Model file for the job. Use its own axes, mm. A direction names the side the tool comes from. Give positions to 0.01 mm unless a question says otherwise; leave off trailing zeros. Loops run counter-clockwise (first coordinate to the right, second up) from the corner with the lowest first, then second, coordinate; pieces in that order, holes last. Notation, with made-up numbers: M 75.25,-37.5 L 84.25,-37.5 A32 cw 84.25,-1.5 Z; hole C 19.25,46 d2. An arc over 180 degrees is marked long. Answer in a Markdown table with one row per item.
Autodesk Inventor part; units mm, degrees
ref_plane "YZ Plane" through (0, 0, 0) normal (1, 0, 0) x (0, 1, 0)
ref_plane "XZ Plane" through (0, 0, 0) normal (0, 1, 0) x (-1, 0, 0)
ref_plane "XY Plane" through (0, 0, 0) normal (0, 0, 1) x (1, 0, 0)
sketch "スケッチ1" plane through (0, 0, 0) normal (0, 1, 0) x (-1, 0, 0)
  line L0 (12.5, 12.5) -> (-12.5, 12.5)
  line L1 (-12.5, 12.5) -> (-12.5, -12.5)
  line L2 (-12.5, -12.5) -> (12.5, -12.5)
  line L3 (12.5, -12.5) -> (12.5, 12.5)
  line L4 (12.5, 12.5) -> (-12.5, -12.5) construction
  line L5 (-12.5, 12.5) -> (12.5, -12.5) construction
  point P0 (0, 0)
  dimension "d0" = 25
  dimension "d1" = 25
extrude "押し出し1" add sketch "スケッチ1" along normal blind 60
shell "シェル1" thickness 2.3 removed faces 2 at (4.1667, 0, -4.1667) at (4.1667, 60, -4.1667)
sketch "スケッチ2" plane through (12.5, 0, 12.5) normal (1, 0, 0) x (0, 0, -1)
  circle A0 centre (12.5, 13) radius 7.5
  line L0 (0, 0) -> (25, 0)
  point P0 (12.5, 0)
  dimension "d5" = 13
  dimension "d6" = 15
extrude "押し出し2" cut sketch "スケッチ2" against normal through all
sketch "スケッチ3" plane through (-12.5, 0, 12.5) normal (0, 0, 1) x (1, 0, 0)
  line L0 (0, 60) -> (25, 60)
  line L1 (2.3, 60) -> (22.7, 60)
  line L2 (22.7, 60) -> (22.7, 40)
  line L3 (22.7, 40) -> (2.3, 40)
  line L4 (2.3, 40) -> (2.3, 60)
  line L5 (0, 0) -> (0, 60)
  line L6 (25, 0) -> (25, 60)
  point P0 (12.5, 0)
  dimension "d9" = 2.3
  dimension "d10" = 2.3
  dimension "d11" = 20
extrude "押し出し3" cut sketch "スケッチ3" against normal through all
sketch "スケッチ4" plane through (12.5, 0, 12.5) normal (1, 0, 0) x (0, 0, -1)
  circle A0 centre (12.5, 50) radius 4
  line L0 (0, 60) -> (25, 60)
  point P0 (12.5, 0)
  dimension "d14" = 8
  dimension "d15" = 10
extrude "押し出し4" cut sketch "スケッチ4" against normal through all
equation "\"d1\" = d0"
equation "\"d10\" = d9"
properties part number "pipe_square_back" material "鉄、可鍛鉄"
(1) Mould opens along Z. For faces 4 (the flat face through (-10.2, 36, 0)), 5 (the flat face through (11, 60, 0)), 6 (the flat face through (0, 23, -12.5)), 7 (the cylindrical face through (-11.33, 5.68, 1.63)) say: pulls with the +Z half, pulls with the -Z half, needs draft (parallel to the pull), parting line crosses it, or undercut.
Established:
| item | result |
|---|---|
| face 4 | undercut |
| face 5 | needs draft |
| face 6 | pulls with the -Z half |
| face 7 | undercut |
(2) Saw through at C-C, the plane z = 9. Give the cut face in (x, y), and give its area (3 significant figures).
Established:
| item | result |
|---|---|
| outline | M -12.5,0 L -10.2,0 L -10.2,60 L -12.5,60 Z; M 10.2,0 L 12.5,0 L 12.5,60 L 10.2,60 Z |
| area | 276 mm2 |
(3) Saw through at B-B, the plane x = -8.25. Give the cut face in (y, z), and give its area (3 significant figures).
Established:
| item | result |
|---|---|
| outline | M 0,-12.5 L 40,-12.5 L 40,-10.2 L 0,-10.2 Z; M 0,10.2 L 40,10.2 L 40,12.5 L 0,12.5 Z |
| area | 184 mm2 |
(4) Flat gauge pins, fed straight in: P1, Ø4, axis at x = -8, z = 6, coming from the -Y side; P2, Ø0.7, axis at x = 4.5, z = 11.5, coming from the +Y side. Where does each tip first touch, or does it go through?
Established:
| item | result |
|---|---|
| P1 | passes through |
| P2 | stops at y = 40 |
(5) Wall check: L1, parallel to Y at x = -11.4, z = 0; L2, parallel to X at y = 3, z = 6. Give the ranges that are in metal, low to high.
Established:
| item | result |
|---|---|
| L1 | y = 0 to 5.5, 20.5 to 46, 54 to 60 |
| L2 | x = -12.5 to -10.2, 10.2 to 12.5 |
(6) Saw through at A-A, the plane y = 50. Give the cut face in (x, z).
Established:
| item | result |
|---|---|
| outline | M -12.5,-12.5 L -10.2,-12.5 L -10.2,-4 L -12.5,-4 Z; M -12.5,4 L -10.2,4 L -10.2,12.5 L -12.5,12.5 Z; M 10.2,-12.5 L 12.5,-12.5 L 12.5,-4 L 10.2,-4 Z; M 10.2,4 L 12.5,4 L 12.5,12.5 L 10.2,12.5 Z |
(7) Which spindle directions (+Z, -Z, +X, -X, +Y, -Y) get a long thin tool onto all of the face, cutting with end or side? Do faces 1 (the flat face through (0, 40, -11)), 2 (the flat face through (-12.5, 30, 0)), 3 (the flat face through (0, 20, 10.2)). Say none if no direction does.
Established:
| item | result |
|---|---|
| face 1 | +Z, -Z, +Y |
| face 2 | +Z, -Z, -X, +Y, -Y |
| face 3 | +Y, -Y |
(8) Saw through at D-D, the plane y = 13. Give the cut face in (x, z).
Established:
| item | result |
|---|---|
| outline | M -12.5,-12.5 L 12.5,-12.5 L 12.5,-7.5 L 10.2,-7.5 L 10.2,-10.2 L -10.2,-10.2 L -10.2,-7.5 L -12.5,-7.5 Z; M -12.5,7.5 L -10.2,7.5 L -10.2,10.2 L 10.2,10.2 L 10.2,7.5 L 12.5,7.5 L 12.5,12.5 L -12.5,12.5 Z |
